Work out the finished part from the listing and answer in its coordinate system (mm). A direction names the side the tool comes from. Give positions to 0.01 mm unless a question says otherwise; leave off trailing zeros. Loops run counter-clockwise (first coordinate to the right, second up) from the corner with the lowest first, then second, coordinate; pieces in that order, holes last. Notation, with made-up numbers: (65, 36) - (112, 36) arc R22 ccw to (112, 71) - close; hole circle Ø7 at (0, 50). An arc over 180 degrees is marked (long way). One line per question, with ' | ' between items.
from build123d import *

# Parameters (mm, degrees)
SKETCH1_W           = 62.23
SKETCH1_H           = 29.21
BOSS_EXTRUDE1_DEPTH = 39.37
SHELL1_T            = -2.54
BOSS_EXTRUDE2_REACH = 31.21


with BuildPart() as part:
    # Sketch1 → Boss-Extrude1 (new body)
    with BuildSketch(Plane.XY):
        with Locations((31.115, 14.605)):
            Rectangle(SKETCH1_W, SKETCH1_H)
    extrude(amount=-BOSS_EXTRUDE1_DEPTH)

    # Shell1
    shell1_openings = [part.faces().sort_by_distance(p)[0] for p in [
        (31.115, 29.21, -19.685),
    ]]
    offset(amount=SHELL1_T, openings=shell1_openings, kind=Kind.INTERSECTION)

    # Sketch2 → Boss-Extrude2 (add, up to next)
    with BuildSketch(Plane(origin=(0, 29.21, 0), x_dir=(1, 0, 0), z_dir=(0, 1, 0)), mode=Mode.PRIVATE) as boss_extrude2_sk1:
        with BuildLine():
            Line((2.54, 2.54), (4.0005, 2.54))
            ThreePointArc((4.0005, 2.54), (2.967770546, 2.967770546), (2.54, 4.0005))
            Line((2.54, 4.0005), (2.54, 2.54))
        make_face()
    boss_extrude2_tool1 = extrude(boss_extrude2_sk1.sketch, amount=-BOSS_EXTRUDE2_REACH, mode=Mode.PRIVATE) - part.part
    add(boss_extrude2_tool1.solids().sort_by_distance((2.866229, 29.21, -2.866229))[0])
    # Sketch2 → Boss-Extrude2 (add, up to next)
    with BuildSketch(Plane(origin=(0, 29.21, 0), x_dir=(1, 0, 0), z_dir=(0, 1, 0)), mode=Mode.PRIVATE) as boss_extrude2_sk2:
        with BuildLine():
            ThreePointArc((58.2295, 36.83), (59.262229454, 36.402229454), (59.69, 35.3695))
            Line((59.69, 35.3695), (59.69, 36.83))
            Line((59.69, 36.83), (58.2295, 36.83))
        make_face()
    boss_extrude2_tool2 = extrude(boss_extrude2_sk2.sketch, amount=-BOSS_EXTRUDE2_REACH, mode=Mode.PRIVATE) - part.part
    add(boss_extrude2_tool2.solids().sort_by_distance((59.363771, 29.21, -36.503771))[0])
    # Sketch2 → Boss-Extrude2 (add, up to next)
    with BuildSketch(Plane(origin=(0, 29.21, 0), x_dir=(1, 0, 0), z_dir=(0, 1, 0)), mode=Mode.PRIVATE) as boss_extrude2_sk3:
        with BuildLine():
            Line((55.88, 33.02), (59.69, 33.02))
            Line((59.69, 33.02), (59.69, 35.3695))
            ThreePointArc((59.69, 35.3695), (57.196770546, 34.336770546), (58.2295, 36.83))
            Line((58.2295, 36.83), (55.88, 36.83))
            Line((55.88, 36.83), (55.88, 33.02))
        make_face()
    boss_extrude2_tool3 = extrude(boss_extrude2_sk3.sketch, amount=-BOSS_EXTRUDE2_REACH, mode=Mode.PRIVATE) - part.part
    add(boss_extrude2_tool3.solids().sort_by_distance((57.05475, 29.21, -36.776118))[0])
    # Sketch2 → Boss-Extrude2 (add, up to next)
    with BuildSketch(Plane(origin=(0, 29.21, 0), x_dir=(1, 0, 0), z_dir=(0, 1, 0)), mode=Mode.PRIVATE) as boss_extrude2_sk4:
        with BuildLine():
            Line((4.0005, 2.54), (6.35, 2.54))
            Line((6.35, 2.54), (6.35, 6.35))
            Line((6.35, 6.35), (2.54, 6.35))
            Line((2.54, 6.35), (2.54, 4.0005))
            ThreePointArc((2.54, 4.0005), (4.0005, 5.461), (5.461, 4.0005))
            ThreePointArc((5.461, 4.0005), (5.033229454, 2.967770546), (4.0005, 2.54))
        make_face()
    boss_extrude2_tool4 = extrude(boss_extrude2_sk4.sketch, amount=-BOSS_EXTRUDE2_REACH, mode=Mode.PRIVATE) - part.part
    add(boss_extrude2_tool4.solids().sort_by_distance((4.0005, 29.21, -5.514882))[0])


solid = part.part
1. Find section C-C on x = 47.5. Write down the section's boundary in (y, z), then the cut area to 3 significant figures.
Evaluation:
outline: (0, -39.37) - (29.21, -39.37) - (29.21, -36.83) - (2.54, -36.83) - (2.54, -2.54) - (29.21, -2.54) - (29.21, 0) - (0, 0) - close | area: 235 mm2
2. Find section B-B on z = -14.5. Write down the section's boundary in (x, y).
Evaluation:
outline: (0, 0) - (62.23, 0) - (62.23, 29.21) - (59.69, 29.21) - (59.69, 2.54) - (2.54, 2.54) - (2.54, 29.21) - (0, 29.21) - close
3. Find section A-A on y = 23.75. Write down the section's boundary in (x, z), then the cut area to 3 significant figures.
Evaluation:
outline: (0, -39.37) - (62.23, -39.37) - (62.23, 0) - (0, 0) - close; hole (2.54, -36.83) - (55.88, -36.83) - (55.88, -33.02) - (59.69, -33.02) - (59.69, -2.54) - (6.35, -2.54) - (6.35, -6.35) - (2.54, -6.35) - close; hole circle Ø2.92 at (4, -4); hole circle Ø2.92 at (58.23, -35.37) | area: 506 mm2
4. Which of the six approach directions +Z, -Z, +X, -X, +Y, -Y give full straight-line access (tool end or side, diameter ignored) to faces 5 (the flat face through (29, 29.21, -2)), 6 (the flat face through (33, 16, -2.54))?
Evaluation:
face 5: +Z, -Z, +X, -X, +Y | face 6: +Y
5. Determine the mould class of faces 1 (the flat face through (62.23, 14, -19)), 2 (the flat face through (31, 15, 0)), 3 (the flat face through (4, 2.54, -4)), 4 (the flat face through (2.54, 16, -21)) for opening direction X: +X half, -X half, draft (parallel to the pull), parting line (faces both ways), or undercut.
Evaluation:
face 1: +X half | face 2: draft | face 3: undercut | face 4: undercut
6. A flat-ended cylindrical pin translates along its axis: pin 1 (8 mm diameter, centred on x = 8, z = -27, fed in from +Y). Find the tip coordinate at first contact, or state that the pin passes through.
Evaluation:
pin 1: y = 2.54
7. Consider L1, parallel to Z at x = 4, y = 13.5; L2, parallel to X at y = 11.5, z = -24.5; L3, parallel to Z at x = 51.5, y = 25.75. Determine where each line is inside the solid, lowest interval first.
Evaluation:
L1: -39.37 to -36.83, -6.35 to -5.46, -2.54 to 0 | L2: 0 to 2.54, 59.69 to 62.23 | L3: -39.37 to -36.83, -2.54 to 0
